from build123d import *

# Parameters (mm, degrees)
BOSS_EXTRUDE1_DEPTH = 40
SKETCH3_W           = 36
SKETCH3_H           = 38
CUT_EXTRUDE1_DEPTH  = 36
CUT_EXTRUDE2_REACH  = 70.147
SKETCH4_R           = 3


with BuildPart() as part:
    # Sketch1 → Boss-Extrude1 (new body)
    with BuildSketch(Plane(origin=(0, 0, 0), x_dir=(0, 0, -1), z_dir=(1, 0, 0))):
        Polygon((0, 0), (0, 40), (40, 0), align=None)
    extrude(amount=BOSS_EXTRUDE1_DEPTH)

    # Sketch3 → Cut-Extrude1 (cut)
    with BuildSketch(Plane.XY.offset(-40)):
        with Locations((20, 21)):
            Rectangle(SKETCH3_W, SKETCH3_H)
    extrude(amount=CUT_EXTRUDE1_DEPTH, mode=Mode.SUBTRACT)

    # Sketch4 → Cut-Extrude2 (cut, up to next)
    with BuildSketch(Plane(origin=(0, 2, 0), x_dir=(1, 0, 0), z_dir=(0, 1, 0)), mode=Mode.PRIVATE) as cut_extrude2_sk1:
        with Locations(Location((20, 21, 0), (0, 0, 270))):
            Circle(SKETCH4_R)
    cut_extrude2_tool1 = extrude(cut_extrude2_sk1.sketch, amount=-CUT_EXTRUDE2_REACH, mode=Mode.PRIVATE) & part.part
    add(cut_extrude2_tool1.solids().sort_by_distance((20, 2, -21))[0], mode=Mode.SUBTRACT)


solid = part.part
Input: part model. Units: mm. Frame: model coordinates. A direction names the side the tool comes from. Round coordinates to 2 decimals unless told otherwise and drop trailing zeros. Write each loop counter-clockwise with the first axis right and the second up, starting at its lowest first coordinate (ties: lowest second). Pieces come first, ordered by that corner, then holes.
1) Cut plane C-C (y = 4). Return the cut outline in (x, z), then the cut area to 3 significant figures.
2) Contact query for a flat-ended pin moving along its axis: P1, Ø2, axis at x = 19, z = -9, coming from the -Y side. Output: stop coordinate, or through.
3) Cut plane A-A (z = -21). Return the cut outline in (x, y).
4) Ray query, L1, parallel to X at y = 33.5, z = -4.5; L2, parallel to X at y = 1.2, z = -21; L3, parallel to Y at x = 12.5, z = -27. Return the intervals inside material, ascending.
5) Cut plane D-D (z = -16). Return the cut outline in (x, y).
6) Cut plane B-B (x = 20). Return the cut outline in (y, z), then the cut area to 3 significant figures.
7) Draft query along X for faces 3 (the flat face through (20, 20, 0)), 4 (the flat face through (38, 11, -14)), 5 (the flat face through (0, 11, -11)). Return one class per face: pulls with the +X half, pulls with the -X half, needs draft (parallel to the pull), parting line crosses it, or undercut.
8) Reachability of faces 1 (the flat face through (2, 11, -14)), 2 (the flat face through (20, 0, -25)) from +Z, -Z, +X, -X, +Y, -Y: full face, straight path, thin tool, end or side. Return the list, or none.
Geometry says:
1. outline: (0, -36) - (2, -36) - (2, -4) - (38, -4) - (38, -36) - (40, -36) - (40, 0) - (0, 0) - close
1. area: 288 mm2
2. P1: stops at y = 0
3. outline: (0, 0) - (17, 0) - (17, 2) - (2, 2) - (2, 19) - (0, 19) - close; (23, 0) - (40, 0) - (40, 19) - (38, 19) - (38, 2) - (23, 2) - close
4. L1: x = 0 to 2, 38 to 40
4. L2: x = 0 to 17, 23 to 40
4. L3: y = 0 to 2
5. outline: (0, 0) - (40, 0) - (40, 24) - (38, 24) - (38, 2) - (2, 2) - (2, 24) - (0, 24) - close
6. outline: (0, -40) - (2, -38) - (2, -24) - (0, -24) - close; (0, -18) - (2, -18) - (2, -4) - (36, -4) - (40, 0) - (0, 0) - close
6. area: 210 mm2
7. face 3: needs draft
7. face 4: undercut
7. face 5: pulls with the -X half
8. face 1: -Z, +Y
8. face 2: +Z, -Z, +X, -X, -Y
